```python
from build123d import *

# Parameters (mm, degrees)
SKETCH_1_R          = 2.5
SKETCH_1_R_2        = 1.8
EXTRUDE_1_DEPTH     = 16
CUT_EXTRUDE_1_REACH = 33.357
SKETCH_2_W          = 8
SKETCH_2_H          = 10


with BuildPart() as part:
    # 草图1 → 凸台-拉伸1 (new body)
    # profile 1 of 3: a face of its own
    with BuildSketch(Plane(origin=(0, 0, 0), x_dir=(1, 0, 0), z_dir=(0, 1, 0))):
        with BuildLine():
            Line((24, -1.5), (4, -1.5))
            ThreePointArc((4, -1.5), (5.767766953, -2.232233047), (6.5, -4))
            ThreePointArc((6.5, -4), (5.767766953, -5.767766953), (4, -6.5))
            Line((4, -6.5), (24, -6.5))
            ThreePointArc((24, -6.5), (21.5, -4), (24, -1.5))
        make_face()
    # profile 2 of 3: a face of its own
    with BuildSketch(Plane(origin=(0, 0, 0), x_dir=(1, 0, 0), z_dir=(0, 1, 0))):
        with Locations((4, -4)):
            Circle(SKETCH_1_R)
        with Locations(Location((4, -4, 0), (0, 0, 270))):
            Circle(SKETCH_1_R_2, mode=Mode.SUBTRACT)
    # profile 3 of 3: a face of its own
    with BuildSketch(Plane(origin=(0, 0, 0), x_dir=(1, 0, 0), z_dir=(0, 1, 0))):
        with Locations((24, -4)):
            Circle(SKETCH_1_R)
        with Locations(Location((24, -4, 0), (0, 0, 270))):
            Circle(SKETCH_1_R_2, mode=Mode.SUBTRACT)
    extrude(amount=EXTRUDE_1_DEPTH)

    # 草图2 → 切除-拉伸1 (cut, up to next)
    with BuildSketch(Plane.XY.offset(6.5), mode=Mode.PRIVATE) as cut_extrude_1_sk1:
        with Locations((22.5, 8)):
            Rectangle(SKETCH_2_W, SKETCH_2_H)
    cut_extrude_1_tool1 = extrude(cut_extrude_1_sk1.sketch, amount=-CUT_EXTRUDE_1_REACH, mode=Mode.PRIVATE) & part.part
    # 草图2 → 切除-拉伸1 (cut, up to next)
    with BuildSketch(Plane.XY.offset(6.5), mode=Mode.PRIVATE) as cut_extrude_1_sk2:
        with Locations((5.5, 8)):
            Rectangle(SKETCH_2_W, SKETCH_2_H)
    cut_extrude_1_tool2 = extrude(cut_extrude_1_sk2.sketch, amount=-CUT_EXTRUDE_1_REACH, mode=Mode.PRIVATE) & part.part
    add(cut_extrude_1_tool1.solids().sort_by_distance((22.5, 8, 6.5))[0], mode=Mode.SUBTRACT)
    add(cut_extrude_1_tool2.solids().sort_by_distance((5.5, 8, 6.5))[0], mode=Mode.SUBTRACT)


solid = part.part
```
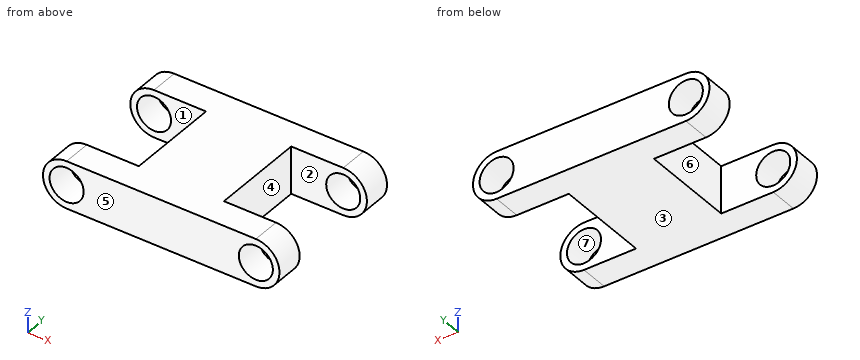
The model under review builds one solid part; all positions refer to its coordinate system, in mm. Face numbers are marked on the shaded views. A direction names the side the tool comes from. Round coordinates to 2 decimals unless told otherwise and drop trailing zeros. Loops run counter-clockwise (first coordinate to the right, second up) from the corner with the lowest first, then second, coordinate; pieces in that order, holes last. Notation, with made-up numbers: M -39,72 L -15,72 A24 ccw -15,94 Z; hole C 36,89.25 d10. An arc over 180 degrees is marked long. Answer as a JSON object with one key per item and string values.
(1) Clearance check with flat-ended pins moving along their axes: P1, Ø2.5, axis at y = 10, z = 4.5, coming from the -X side; P2, Ø3, axis at y = 12.5, z = 2.5, coming from the +X side. State where each tip first meets the part, or that it passes through.
Resolved:
{"P1": "x = 9.5", "P2": "x = 26.5"}
(2) To check wall thickness, follow line 1 along X through (y, z) = (1.15, 4); line 2 along Y through (x, z) = (20.5, 4.15); line 3 along X through (y, z) = (2.25, 3). State the ranges of each line that lie inside material, in increasing order.
Resolved:
{"line 1": "1.5 to 2.2, 5.8 to 22.2, 25.8 to 26.5", "line 2": "0 to 3, 13 to 16", "line 3": "1.71 to 2.5, 5.5 to 22.5, 25.5 to 26.29"}
(3) Draft analysis for pull direction X (two halves, no side actions). For the marked faces 4, 5, 6 and 7, state which applies: released by +X, released by -X, zero draft, split by the parting line, or undercut.
Resolved:
{"face 4": "released by +X", "face 5": "zero draft", "face 6": "released by -X", "face 7": "undercut"}
(4) Tool access review of the marked faces 1, 2 and 3: name each direction out of +Z, -Z, +X, -X, +Y, -Y from which nothing blocks a thin tool from reaching the whole face with its end or side.
Resolved:
{"face 1": "+Z, -Z, -X", "face 2": "+Z, -Z, +X", "face 3": "-Z, +X, -X, +Y, -Y"}
(5) Take a section at B-B on x = 21. Give the boundary of the cut face in (y, z), and give its area (3 significant figures).
Resolved:
{"outline": "M 0,1.5 L 3,1.5 L 3,6.5 L 0,6.5 Z; M 13,1.5 L 16,1.5 L 16,6.5 L 13,6.5 Z", "area": "30.0 mm²"}
(6) Take a section at D-D on x = 3.75. Give the boundary of the cut face in (y, z), and give its area (3 significant figures).
Resolved:
{"outline": "M 0,1.51 L 3,1.51 L 3,2.22 L 0,2.22 Z; M 0,5.78 L 3,5.78 L 3,6.49 L 0,6.49 Z; M 13,1.51 L 16,1.51 L 16,2.22 L 13,2.22 Z; M 13,5.78 L 16,5.78 L 16,6.49 L 13,6.49 Z", "area": "8.46 mm²"}
(7) Take a section at A-A on z = 4. Give the boundary of the cut face in (x, y), and give its area (3 significant figures).
Resolved:
{"outline": "M 1.5,0 L 2.2,0 L 2.2,3 L 1.5,3 Z; M 1.5,13 L 2.2,13 L 2.2,16 L 1.5,16 Z; M 5.8,0 L 22.2,0 L 22.2,3 L 18.5,3 L 18.5,13 L 22.2,13 L 22.2,16 L 5.8,16 L 5.8,13 L 9.5,13 L 9.5,3 L 5.8,3 Z; M 25.8,0 L 26.5,0 L 26.5,3 L 25.8,3 Z; M 25.8,13 L 26.5,13 L 26.5,16 L 25.8,16 Z", "area": "197 mm²"}
(8) Take a section at C-C on y = 14.25. Give the boundary of the cut face in (x, z), and give its area (3 significant figures).
Resolved:
{"outline": "M 4,1.5 L 24,1.5 A2.5 ccw 24,6.5 L 4,6.5 A2.5 ccw Z; hole C 4,4 d3.6; hole C 24,4 d3.6", "area": "99.3 mm²"}
